The model under review builds one solid part; all positions refer to its coordinate system, in mm. A direction names the side the tool comes from. Round coordinates to 2 decimals unless told otherwise and drop trailing zeros. Loops run counter-clockwise (first coordinate to the right, second up) from the corner with the lowest first, then second, coordinate; pieces in that order, holes last. Notation, with made-up numbers: M 53.25,70.5 L 97.25,70.5 A12 cw 97.25,85.5 Z; hole C 85.25,70 d10. An arc over 180 degrees is marked long. Answer as a JSON object with one key per item and string values. Group by question number.
Item 1: Consider section A-A (x = 9.5). Give the boundary of the cut face in (y, z), and give its area (3 significant figures).
Item 2: Insertion check: P1, Ø12, axis at y = 22, z = 20.5, coming from the +X side; P2, Ø7.5, axis at y = 41, z = 15, coming from the +X side; P3, Ø3, axis at x = 43, y = 33, coming from the -Z side; P4, Ø3.5, axis at x = 1, z = 9.5, coming from the -Y side. Each pin has a flat end and moves straight along its axis. Give the tip position at first contact, or say it passes through.
Item 3: The part is to be moulded in two halves that separate along X. For faces 1 (the face through (55, 17, 15)), 2 (the face through (28.704, 51.844, 15.21)), 3 (the face through (3.6, 51.43, 15.21)), 4 (the face through (0, 44, 15)), say which applies: +X half, -X half, draft (parallel to the pull), parting line (faces both ways), or undercut.
Item 4: Consider section B-B (z = 16). State how many separate pieces and enclosed holes the cut face has, and give its area (3 significant figures).
Item 5: To check wall thickness, follow line 1 (Y direction, x = 1.75, z = 15); line 2 (X direction, y = 0.9, z = 15); line 3 (Y direction, x = 10, z = 20.5). State the ranges of each line that lie inside material, in increasing order.
Item 6: Consider section C-C (z = 25.5). Give the boundary of the cut face in (x, y).
Item 7: Consider section D-D (y = 41). Give the boundary of the cut face in (x, z), and give its area (3 significant figures).
Item 8: Tool access review of faces 5 (the face through (47, 34, 0)), 6 (the face through (51.4, 3.57, 15.21)), 7 (the face through (66, 3, 15)): name each direction out of +Z, -Z, +X, -X, +Y, -Y from which nothing blocks a thin tool from reaching the whole face with its end or side.
```python
from build123d import *

# Parameters (mm, degrees)
EXTRUDE_THIN1_DEPTH  = 30
M4_CLEARANCE_HOLE1_D = 4.8
M4_CLEARANCE_HOLE2_D = 4.8
FILLET1_R            = 1
FILLET2_R            = 2


# Read off the part's stored shape, not the designer's step: Extrude-Thin1
with BuildPart() as part:
    # Extrude-Thin1 outline → Extrude-Thin1 (new body)
    with BuildSketch(Plane.XY):
        Polygon((0, 3), (0, 0), (70, 0), (70, 3), (55, 3), (55, 30), (30, 55), (0, 55), (0, 35), (3, 35), (3, 52), (28.757359313, 52), (52, 28.757359313), (52, 3), align=None)
    extrude(amount=EXTRUDE_THIN1_DEPTH)

    # M4 Clearance Hole1 (through all)
    with Locations(Plane.ZY):
        with Locations((15, 41)):
            Hole(M4_CLEARANCE_HOLE1_D / 2)

    # M4 Clearance Hole2 (through all)
    with Locations(Plane(origin=(0, 3, 0), x_dir=(1, 0, 0), z_dir=(0, 1, 0))):
        with Locations((62.5, -15)):
            Hole(M4_CLEARANCE_HOLE2_D / 2)

    # Fillet1
    fillet1_edges = [part.edges().sort_by_distance(p)[0] for p in [
        (1.5, 35, 0),
        (1.5, 35, 30),
        (0, 1.5, 0),
        (0, 1.5, 30),
        (70, 1.5, 0),
        (70, 1.5, 30),
    ]]
    fillet(fillet1_edges, radius=FILLET1_R)

    # Fillet2
    fillet2_edges = [part.edges().sort_by_distance(p)[0] for p in [
        (0, 55, 15),
        (30, 55, 15),
        (55, 30, 15),
        (52, 28.757359313, 15),
        (28.757359313, 52, 15),
        (3, 52, 15),
        (55, 3, 15),
        (52, 3, 15),
    ]]
    fillet(fillet2_edges, radius=FILLET2_R)


solid = part.part
```
Geometry results:
{
 "1": {"outline": "M 0,0 L 3,0 L 3,30 L 0,30 Z; M 52,0 L 55,0 L 55,30 L 52,30 Z", "area": "180 mm^2"},
 "2": {"P1": "stops at x = 55", "P2": "stops at x = 47.75", "P3": "passes through", "P4": "stops at y = 0"},
 "3": {"face 1": "+X half", "face 2": "undercut", "face 3": "undercut", "face 4": "-X half"},
 "4": {"separate pieces": "4", "enclosed holes": "0", "area": "488 mm^2"},
 "5": {"line 1": "y = 0 to 3, 35 to 38.6, 43.4 to 54.98", "line 2": "x = 0 to 60.1, 64.9 to 70", "line 3": "y = 0 to 3, 52 to 55"},
 "6": {"outline": "M 0,0 L 70,0 L 70,3 L 57,3 A2 cw 55,5 L 55,29.17 A2 ccw 54.41,30.59 L 30.59,54.41 A2 ccw 29.17,55 L 2,55 A2 ccw 0,53 L 0,35 L 3,35 L 3,50 A2 cw 5,52 L 27.93,52 A2 cw 29.34,51.41 L 51.41,29.34 A2 cw 52,27.93 L 52,5 A2 cw 50,3 L 0,3 Z"},
 "7": {"outline": "M 0,0 L 3,0 L 3,12.6 L 0,12.6 Z; M 0,17.4 L 3,17.4 L 3,30 L 0,30 Z; M 39.76,0 L 44,0 L 44,12.6 L 39.76,12.6 Z; M 39.76,17.4 L 44,17.4 L 44,30 L 39.76,30 Z", "area": "183 mm^2"},
 "8": {"face 5": "-Z, +X, -X, +Y, -Y", "face 6": "+Z, -Z, -X", "face 7": "+Z, -Z, +X, +Y"}
}
